Source: CAD feature listing. Evaluate the final solid. Frame: model axes, mm. Face numbers are marked on the shaded views. A direction names the side the tool comes from. Give positions to 0.01 mm unless a question says otherwise; leave off trailing zeros. Order: outer loops, then holes, each group sorted by start corner. A loop starts at its lowest first (then second) coordinate and runs counter-clockwise, first axis right, second up.
```python
from build123d import *

# Parameters (mm, degrees)
F0_R     = 1.5
F1_DEPTH = 5
F2_R     = 2.75
F3_DEPTH = 2.5
F5_DEPTH = 1.5
F6_SIZE  = 0.25


with BuildPart() as f1:
    # F0 (on Top) → F1 (new body)
    with BuildSketch(Plane.XY):
        Circle(F0_R)
    extrude(amount=F1_DEPTH)

    # F2 (on face) → F3 (join)
    with BuildSketch(Plane(origin=(0, 0, 0), x_dir=(1, 0, 0), z_dir=(0, 0, -1))):
        Circle(F2_R)
    extrude(amount=F3_DEPTH)

    # F4 (on face) → F5 (cut)
    with BuildSketch(Plane(origin=(0, 0, -2.5), x_dir=(1, 0, 0), z_dir=(0, 0, -1))):
        Polygon((1.75, -1.010363), (1.75, 1.010363), (0, 2.020726), (-1.75, 1.010363), (-1.75, -1.010363), (0, -2.020726), align=None)
    extrude(amount=-F5_DEPTH, mode=Mode.SUBTRACT)

    # F6
    f6_edges = [f1.edges().sort_by_distance(p)[0] for p in [
        (-2.75, 0, 0),
        (-2.75, 0, -2.5),
    ]]
    chamfer(f6_edges, length=F6_SIZE)


solid = f1.part
```
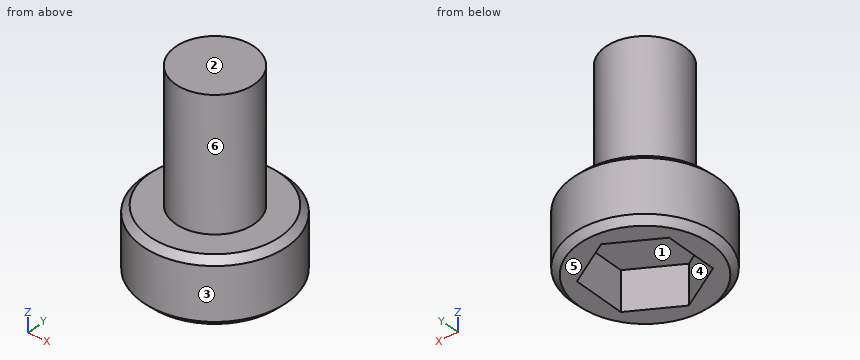
1) Section query C-C, the plane z = 3.5. Return the cut outline in (x, y).
Report:
outline: circle Ø3 at (0, 0)
2) Pin query (flat end, axial travel): pin 1 (2 mm diameter, centred on y = 0, z = 2, fed in from +X); pin 2 (1.5 mm diameter, centred on x = -1.5, z = -1.5, fed in from +Y); pin 3 (1.8 mm diameter, centred on x = -0.5, y = -0.5, fed in from -Z). Return the tip coordinate at first contact, or that it passes through.
Report:
pin 1: stops at x = 1.5
pin 2: stops at y = 2.65
pin 3: stops at z = -1
3) Section query B-B, the plane y = 0. Return the cut outline in (x, z), and give its area (3 significant figures).
Report:
outline: (-2.75, -2.25) - (-2.5, -2.5) - (-1.75, -2.5) - (-1.75, -1) - (1.75, -1) - (1.75, -2.5) - (2.5, -2.5) - (2.75, -2.25) - (2.75, -0.25) - (2.5, 0) - (1.5, 0) - (1.5, 5) - (-1.5, 5) - (-1.5, 0) - (-2.5, 0) - (-2.75, -0.25) - close
area: 23.4 mm2
4) Reachability of the marked faces 4, 5 and 6 from +Z, -Z, +X, -X, +Y, -Y: full face, straight path, thin tool, end or side. Return the list, or none.
Report:
face 4: -Z
face 5: -Z, +X, -X, +Y, -Y
face 6: +Z
5) Draft query along Y for the marked faces 1, 2 and 3. Return one class per face: +Y half, -Y half, draft (parallel to the pull), parting line (faces both ways), or undercut.
Report:
face 1: undercut
face 2: draft
face 3: parting line
6) Section query A-A, the plane z = -2. Return the cut outline in (x, y), and give its area (3 significant figures).
Report:
outline: circle Ø5.5 at (0, 0); hole (-1.75, -1.01) - (0, -2.02) - (1.75, -1.01) - (1.75, 1.01) - (0, 2.02) - (-1.75, 1.01) - close
area: 13.1 mm2
7) Material intervals for L1, parallel to Z at x = 0.4, y = -0.45; L2, parallel to Z at x = -0.75, y = 2.3; L3, parallel to Y at x = 0.5, z = -1.25, sorted ascending.
Report:
L1: z = -1 to 5
L2: z = -2.5 to 0
L3: y = -2.7 to -1.73, 1.73 to 2.7
